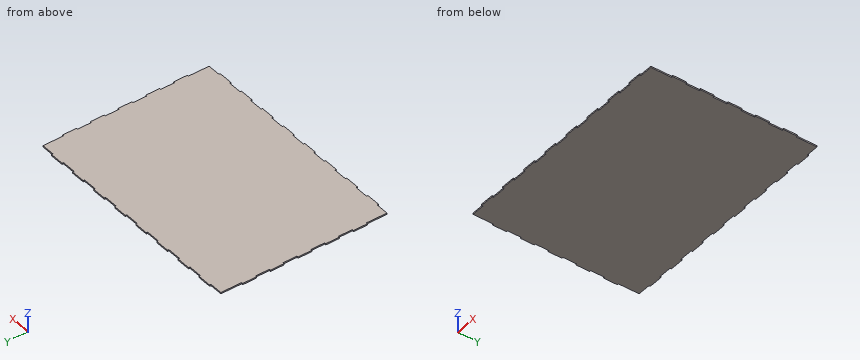
from build123d import *

# Parameters (mm, degrees)
BOSS_EXTRUDE1_DEPTH = 50
SCALE1_SCALE        = 0.04


with BuildPart() as part:
    # Sketch1 → Boss-Extrude1 (new body)
    with BuildSketch(Plane.XY):
        Polygon((-1.484062936, 0.145079086), (487.465937064, 0.145079086), (487.465937064, -50.654920914), (1008.165937064, -50.654920914), (1008.165937064, 0.145079086), (1528.865937064, 0.145079086), (1528.865937064, -50.654920914), (2049.565937064, -50.654920914), (2049.565937064, 0.145079086), (2570.265937064, 0.145079086), (2570.265937064, -50.654920914), (3090.965937064, -50.654920914), (3090.965937064, 0.145079086), (3611.665937064, 0.145079086), (3611.665937064, -50.654920914), (4132.365937064, -50.654920914), (4132.365937064, 0.145079086), (4653.065937064, 0.145079086), (4653.065937064, -50.654920914), (5173.765937064, -50.654920914), (5173.765937064, 0.145079086), (5694.465937064, 0.145079086), (5694.465937064, -50.654920914), (6215.165937064, -50.654920914), (6215.165937064, 0.145079086), (6735.865937064, 0.145079086), (6735.865937064, -50.654920914), (7256.565937064, -50.654920914), (7256.565937064, 0.145079086), (7777.265937064, 0.145079086), (7777.265937064, -50.654920914), (8297.965937064, -50.654920914), (8297.965937064, 0.145079086), (8786.915937064, 0.145079086), (8786.915937064, 781.195079086), (8837.715937064, 781.195079086), (8837.715937064, 1301.895079086), (8786.915937064, 1301.895079086), (8786.915937064, 1822.595079086), (8837.715937064, 1822.595079086), (8837.715937064, 2343.295079086), (8786.915937064, 2343.295079086), (8786.915937064, 2863.995079086), (8837.715937064, 2863.995079086), (8837.715937064, 3384.695079086), (8786.915937064, 3384.695079086), (8786.915937064, 3905.395079086), (8837.715937064, 3905.395079086), (8837.715937064, 4426.095079086), (8786.915937064, 4426.095079086), (8786.915937064, 4946.795079086), (8837.715937064, 4946.795079086), (8837.715937064, 5467.495079086), (8786.915937064, 5467.495079086), (8786.915937064, 5988.195079086), (8786.915937064, 6248.545079086), (8297.965937064, 6248.545079086), (8297.965937064, 6299.345079086), (7777.265937064, 6299.345079086), (7777.265937064, 6248.545079086), (7256.565937064, 6248.545079086), (7256.565937064, 6299.345079086), (6735.865937064, 6299.345079086), (6735.865937064, 6248.545079086), (6215.165937064, 6248.545079086), (6215.165937064, 6299.345079086), (5694.465937064, 6299.345079086), (5694.465937064, 6248.545079086), (5173.765937064, 6248.545079086), (5173.765937064, 6299.345079086), (4653.065937064, 6299.345079086), (4653.065937064, 6248.545079086), (4132.365937064, 6248.545079086), (4132.365937064, 6299.345079086), (3611.665937064, 6299.345079086), (3611.665937064, 6248.545079086), (3090.965937064, 6248.545079086), (3090.965937064, 6299.345079086), (2570.265937064, 6299.345079086), (2570.265937064, 6248.545079086), (2049.565937064, 6248.545079086), (2049.565937064, 6299.345079086), (1528.865937064, 6299.345079086), (1528.865937064, 6248.545079086), (1008.165937064, 6248.545079086), (1008.165937064, 6299.345079086), (487.465937064, 6299.345079086), (487.465937064, 6248.545079086), (-1.484062936, 6248.545079086), (-1.484062936, 5467.495079086), (-52.284062936, 5467.495079086), (-52.284062936, 4946.795079086), (-1.484062936, 4946.795079086), (-1.484062936, 4426.095079086), (-52.284062936, 4426.095079086), (-52.284062936, 3905.395079086), (-1.484062936, 3905.395079086), (-1.484062936, 3384.695079086), (-52.284062936, 3384.695079086), (-52.284062936, 2863.995079086), (-1.484062936, 2863.995079086), (-1.484062936, 2343.295079086), (-52.284062936, 2343.295079086), (-52.284062936, 1822.595079086), (-1.484062936, 1822.595079086), (-1.484062936, 1301.895079086), (-52.284062936, 1301.895079086), (-52.284062936, 781.195079086), (-1.484062936, 781.195079086), (-1.484062936, 260.495079086), align=None)
    extrude(amount=BOSS_EXTRUDE1_DEPTH)


with BuildPart() as part_1:
    # Scale1: scaled about (4392.715937064, 3124.345079086, 25)
    add(part.part.scale(SCALE1_SCALE).moved(Location((4217.007299581, 2999.371275923, 24))))


solid = part_1.part
Check sheet for the modelled part. Datum: model origin and axes. Units: mm. Round coordinates to 2 decimals unless told otherwise and drop trailing zeros. Order: outer loops, then holes, each group sorted by start corner. A loop starts at its lowest first (then second) coordinate and runs counter-clockwise, first axis right, second up. Notation, with made-up numbers: M 4,33 L 25,33 A27 cw 25,64 Z; hole C -9,35 d11. An arc over 180 degrees is marked long. One line per item, written item: value. Start each with the question number.
1. Scan lines: line 1 along Y through (x, z) = (4521, 25.9); line 2 along X through (y, z) = (3221.5, 25.2). Record each from-to range of solid material in increasing order.
2. Gauge pin test, flat ends, axial feed: P1, Ø1, axis at y = 3014.5, z = 25.5, coming from the +X side; P2, Ø0.6, axis at y = 3250, z = 25.5, coming from the +X side; P3, Ø1, axis at y = 3137.5, z = 25.5, coming from the -X side. Record the tip position at first contact, or that the pin passes through.
3. Section check A-A on x = 4349.5. Enter the section's corners in (y, z), and give its area (3 significant figures).
Results found:
1. line 1: 2999.38 to 3249.31
1. line 2: 4216.95 to 4568.48
2. P1: x = 4568.48
2. P2: x = 4548.93
2. P3: x = 4216.95
3. outline: M 2999.38,24 L 3249.31,24 L 3249.31,26 L 2999.38,26 Z
3. area: 500 mm^2
